Design review of the part built by this model. Coordinates are the model's own, in mm. Face numbers are marked on the shaded views. A direction names the side the tool comes from. Coordinates: 2 decimals unless noted, no trailing zeros. Loops run counter-clockwise (first coordinate to the right, second up) from the corner with the lowest first, then second, coordinate; pieces in that order, holes last.
Q1. Add section A-A on z = 19.05. Give the boundary of the cut face in (x, y) (3 decimals).
Q2. Machinability: for the marked faces 1 and 2, which of the approach directions +Z, -Z, +X, -X, +Y, -Y give a long, thin tool a straight path to every point of the face, cutting with its end or side? Answer none if there is none.
Q3. Add section B-B on x = -12.7. Give the boundary of the cut face in (y, z) (3 decimals), and give its area (3 significant figures).
Q4. For P1, Ø3, axis at y = -15.24, z = 12.7, coming from the -X side; P2, Ø3, axis at x = -64.5, z = 38.5, coming from the -Y side (3 decimals); P3, Ø5, axis at y = -20, z = 91, coming from the +X side (3 decimals), all flat-tipped, find the tip position at first contact; note any pin that passes through.
Q5. Add section C-C on z = 38.1. Give the boundary of the cut face in (x, y) (3 decimals).
Q6. Add section D-D on y = -15.24. Give the boundary of the cut face in (x, z) (3 decimals), and give its area (3 significant figures).
Q7. Wall thickness on probe 1 along X at (y, z) = (-2.2, 50.8); probe 2 along Y at (x, z) = (-74.55, 25.4); probe 3 along X at (y, z) = (-20.25, 88.5) (3 decimals): over which ranges is each line inside the solid? List them lowest first.
```python
from build123d import *

# Parameters (mm, degrees)
BOSS_EXTRUDE1_DEPTH       = 76.2
TAP_DRILL_FOR_6_32_TAP1_D = 2.7051
TAP_DRILL_FOR_8_32_TAP1_D = 3.4544
CUT_EXTRUDE1_REACH        = 112.716
SKETCH8_W                 = 3.302
SKETCH8_H                 = 3.302
TAP_DRILL_FOR_8_32_TAP2_D = 3.4544
BOSS_EXTRUDE2_DEPTH       = 50.8


with BuildPart() as part:
    # Sketch2 → Boss-Extrude1 (new body)
    with BuildSketch(Plane.XY):
        Polygon((0, 0), (-76.2, 0), (-76.2, -25.4), (-73.025, -25.4), (-73.025, -3.175), (0, -3.175), align=None)
    extrude(amount=BOSS_EXTRUDE1_DEPTH)

    # Tap Drill for #6-32 Tap1 (through all)
    with Locations(Plane.ZY.offset(76.2)):
        with Locations((25.4, -15.24), (12.7, -15.24)):
            Hole(TAP_DRILL_FOR_6_32_TAP1_D / 2)

    # Tap Drill for #8-32 Tap1 (through all)
    with Locations(Plane(origin=(0, 0, 0), x_dir=(1, 0, 0), z_dir=(0, 1, 0))):
        with Locations((-69.917738612, -25.4), (-69.917738612, -50.8)):
            Hole(TAP_DRILL_FOR_8_32_TAP1_D / 2)

    # Sketch8 → Cut-Extrude1 (cut, up to next)
    with BuildSketch(Plane.ZY.offset(76.2), mode=Mode.PRIVATE) as cut_extrude1_sk1:
        with Locations((38.1, -15.24)):
            Rectangle(SKETCH8_W, SKETCH8_H)
    cut_extrude1_tool1 = extrude(cut_extrude1_sk1.sketch, amount=-CUT_EXTRUDE1_REACH, mode=Mode.PRIVATE) & part.part
    add(cut_extrude1_tool1.solids().sort_by_distance((-76.2, -15.24, 38.1))[0], mode=Mode.SUBTRACT)

    # Tap Drill for #8-32 Tap2 (through all)
    with Locations(Plane(origin=(0, 0, 0), x_dir=(1, 0, 0), z_dir=(0, 1, 0))):
        with Locations((-12.7, -19.05), (-12.7, -38.1), (-12.7, -57.15)):
            Hole(TAP_DRILL_FOR_8_32_TAP2_D / 2)

    # Sketch11 → Boss-Extrude2 (add)
    with BuildSketch(Plane.XY.offset(76.2)):
        Polygon((-76.2, 0), (-76.2, -25.4), (-73.025, -25.4), (-73.025, -3.175), (0, -3.175), (0, 0), align=None)
    extrude(amount=BOSS_EXTRUDE2_DEPTH)


solid = part.part
```
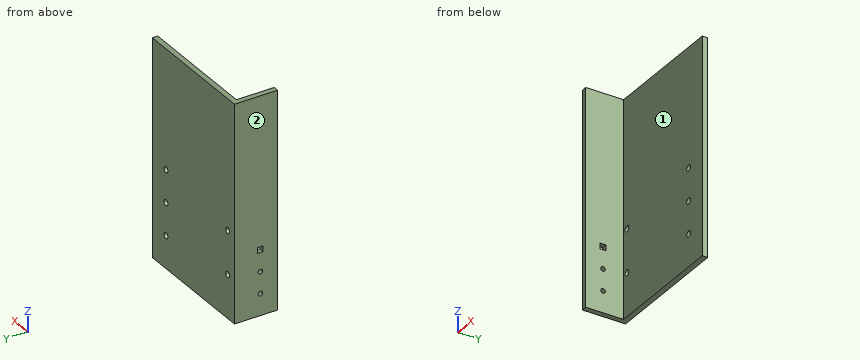
Entries:
1. outline: (-76.2, -25.4) - (-73.025, -25.4) - (-73.025, -3.175) - (-14.427, -3.175) - (-14.427, 0) - (-76.2, 0) - close; (-10.973, -3.175) - (0, -3.175) - (0, 0) - (-10.973, 0) - close
2. face 1: +Z, -Z, +X, -Y
2. face 2: +Z, -Z, -X, +Y, -Y
3. outline: (-3.175, 0) - (0, 0) - (0, 17.323) - (-3.175, 17.323) - close; (-3.175, 20.777) - (0, 20.777) - (0, 36.373) - (-3.175, 36.373) - close; (-3.175, 39.827) - (0, 39.827) - (0, 55.423) - (-3.175, 55.423) - close; (-3.175, 58.877) - (0, 58.877) - (0, 127) - (-3.175, 127) - close
3. area: 370 mm2
4. P1: stops at x = -76.2
4. P2: stops at y = -3.175
4. P3: stops at x = -73.025
5. outline: (-76.2, -25.4) - (-73.025, -25.4) - (-73.025, -16.891) - (-76.2, -16.891) - close; (-76.2, -13.589) - (-73.025, -13.589) - (-73.025, -3.175) - (-14.427, -3.175) - (-14.427, 0) - (-76.2, 0) - close; (-10.973, -3.175) - (0, -3.175) - (0, 0) - (-10.973, 0) - close
6. outline: (-76.2, 0) - (-73.025, 0) - (-73.025, 11.347) - (-76.2, 11.347) - close; (-76.2, 14.053) - (-73.025, 14.053) - (-73.025, 24.047) - (-76.2, 24.047) - close; (-76.2, 26.753) - (-73.025, 26.753) - (-73.025, 36.449) - (-76.2, 36.449) - close; (-76.2, 39.751) - (-73.025, 39.751) - (-73.025, 127) - (-76.2, 127) - close
6. area: 376 mm2
7. probe 1: x = -76.2 to -71.64, -68.19 to 0
7. probe 2: y = -25.4 to -16.59, -13.89 to 0
7. probe 3: x = -76.2 to -73.025
